```python
from build123d import *

# Parameters (mm, degrees)
SKETCH_1_W          = 92
SKETCH_1_H          = 60
EXTRUDE_1_DEPTH     = 1
EXTRUDE_3_DEPTH     = 2
SKETCH_6_W          = 1.8
SKETCH_6_H          = 1.8
CUT_EXTRUDE_3_DEPTH = 1
SKETCH_7_W          = 1.8
SKETCH_7_H          = 1.8
CUT_EXTRUDE_4_DEPTH = 1
SKETCH_8_W          = 1.8
SKETCH_8_H          = 1.8
CUT_EXTRUDE_5_DEPTH = 1
SKETCH_9_W          = 1.8
SKETCH_9_H          = 1.8
CUT_EXTRUDE_6_DEPTH = 1
SKETCH_15_W         = 15
SKETCH_15_H         = 26.7
CUT_EXTRUDE_8_DEPTH = 1


with BuildPart() as part:
    # Эскиз1 → Бобышка-Вытянуть1 (new body)
    with BuildSketch(Plane(origin=(0, 0, 0), x_dir=(1, 0, 0), z_dir=(0, 1, 0))):
        with Locations((46, 30)):
            Rectangle(SKETCH_1_W, SKETCH_1_H)
    extrude(amount=EXTRUDE_1_DEPTH)

    # Эскиз3 → Бобышка-Вытянуть3 (add)
    with BuildSketch(Plane(origin=(0, 1, 0), x_dir=(1, 0, 0), z_dir=(0, 1, 0))):
        Polygon((86, 54), (91, 54), (91, 6), (86, 6), (86, 1), (6, 1), (6, 6), (1, 6), (1, 54), (6, 54), (6, 59), (86, 59), align=None)
        Polygon((7, 58), (7, 53), (2, 53), (2, 7), (7, 7), (7, 2), (85, 2), (85, 7), (90, 7), (90, 53), (85, 53), (85, 58), align=None, mode=Mode.SUBTRACT)
    extrude(amount=EXTRUDE_3_DEPTH)

    # Эскиз6 → Вырез-Вытянуть3 (cut)
    with BuildSketch(Plane(origin=(0, 1, 0), x_dir=(1, 0, 0), z_dir=(0, 1, 0))):
        with Locations((3.5, 56.5)):
            Rectangle(SKETCH_6_W, SKETCH_6_H)
    extrude(amount=-CUT_EXTRUDE_3_DEPTH, mode=Mode.SUBTRACT)

    # Эскиз7 → Вырез-Вытянуть4 (cut)
    with BuildSketch(Plane(origin=(0, 1, 0), x_dir=(1, 0, 0), z_dir=(0, 1, 0))):
        with Locations((88.5, 56.5)):
            Rectangle(SKETCH_7_W, SKETCH_7_H)
    extrude(amount=-CUT_EXTRUDE_4_DEPTH, mode=Mode.SUBTRACT)

    # Эскиз8 → Вырез-Вытянуть5 (cut)
    with BuildSketch(Plane(origin=(0, 1, 0), x_dir=(1, 0, 0), z_dir=(0, 1, 0))):
        with Locations((88.5, 3.5)):
            Rectangle(SKETCH_8_W, SKETCH_8_H)
    extrude(amount=-CUT_EXTRUDE_5_DEPTH, mode=Mode.SUBTRACT)

    # Эскиз9 → Вырез-Вытянуть6 (cut)
    with BuildSketch(Plane(origin=(0, 1, 0), x_dir=(1, 0, 0), z_dir=(0, 1, 0))):
        with Locations((3.5, 3.5)):
            Rectangle(SKETCH_9_W, SKETCH_9_H)
    extrude(amount=-CUT_EXTRUDE_6_DEPTH, mode=Mode.SUBTRACT)

    # Эскиз15 → Вырез-Вытянуть8 (cut)
    with BuildSketch(Plane(origin=(0, 1, 0), x_dir=(1, 0, 0), z_dir=(0, 1, 0))):
        with Locations((46, 30)):
            Rectangle(SKETCH_15_W, SKETCH_15_H)
    extrude(amount=-CUT_EXTRUDE_8_DEPTH, mode=Mode.SUBTRACT)


solid = part.part
```
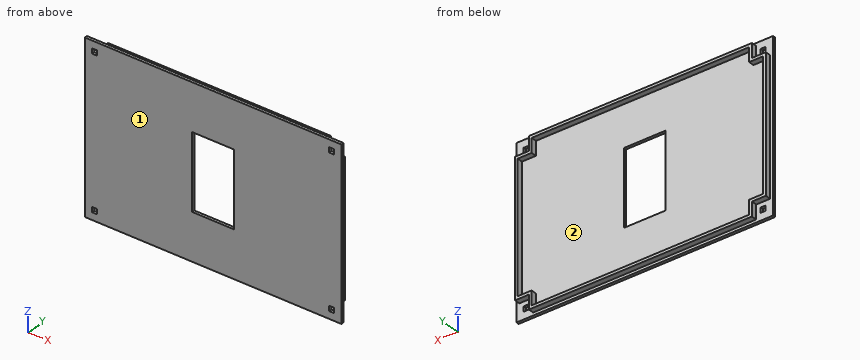
Source: CAD feature listing. Evaluate the final solid. Frame: model axes, mm. Face numbers are marked on the shaded views. Round coordinates to 2 decimals unless told otherwise and drop trailing zeros. Write each loop counter-clockwise with the first axis right and the second up, starting at its lowest first coordinate (ties: lowest second). Pieces come first, ordered by that corner, then holes. Notation, with made-up numbers: M 32,-36.75 L 68,-36.75 A25 ccw 68,-22.75 Z; hole C 12.5,-24 d8. An arc over 180 degrees is marked long. Answer as a JSON object with one key per item and string values. Group by question number.
(1) Section query C-C on y = 2.3. Output: boundary loops of the cut face in (x, z).
(2) First-contact query: pin 1 (18 mm diameter, centred on x = 26.5, z = -40.5, fed in from +Y); pin 2 (1.6 mm diameter, centred on y = 2.5, z = -56.5, fed in from -X). Flat tips, straight axial feed; report the tip coordinate or a pass-through.
(3) Section query D-D on x = 58.5. Output: boundary loops of the cut face in (y, z).
(4) Ray query, line 1 (Z direction, x = 36.5, y = 1.5); line 2 (X direction, y = 2.95, z = -49); line 3 (X direction, y = 0.15, z = -32.5). Return the intervals inside material, ascending. Write a range as [from, to].
(5) Section query B-B on z = -34.5. Output: boundary loops of the cut face in (x, y), then the cut area to 3 significant figures.
(6) Mould query, pull axis Z, two halves, no side actions, for the marked faces 1 and 2. Classes: +Z half, -Z half, draft (parallel to the pull), parting line (faces both ways), or undercut.
(7) Section query A-A on x = 47. Output: boundary loops of the cut face in (y, z).
Computed values:
{
 "1": {"outline": "M 1,-54 L 6,-54 L 6,-59 L 86,-59 L 86,-54 L 91,-54 L 91,-6 L 86,-6 L 86,-1 L 6,-1 L 6,-6 L 1,-6 Z; hole M 2,-53 L 7,-53 L 7,-58 L 85,-58 L 85,-53 L 90,-53 L 90,-7 L 85,-7 L 85,-2 L 7,-2 L 7,-7 L 2,-7 Z"},
 "2": {"pin 1": "y = 1", "pin 2": "x = 6"},
 "3": {"outline": "M 0,-60 L 1,-60 L 1,-59 L 3,-59 L 3,-58 L 1,-58 L 1,-2 L 3,-2 L 3,-1 L 1,-1 L 1,0 L 0,0 Z"},
 "4": {"line 1": "[-59, -58], [-2, -1]", "line 2": "[1, 2], [90, 91]", "line 3": "[0, 38.5], [53.5, 92]"},
 "5": {"outline": "M 0,0 L 38.5,0 L 38.5,1 L 2,1 L 2,3 L 1,3 L 1,1 L 0,1 Z; M 53.5,0 L 92,0 L 92,1 L 91,1 L 91,3 L 90,3 L 90,1 L 53.5,1 Z", "area": "81.0 mm^2"},
 "6": {"face 1": "draft", "face 2": "undercut"},
 "7": {"outline": "M 0,-60 L 1,-60 L 1,-59 L 3,-59 L 3,-58 L 1,-58 L 1,-43.35 L 0,-43.35 Z; M 0,-16.65 L 1,-16.65 L 1,-2 L 3,-2 L 3,-1 L 1,-1 L 1,0 L 0,0 Z"}
}
